Drawing for the job (mm, zero at the part's lowest x, y, z). A direction names the side the tool comes from. Give positions to 0.01 mm unless a question says otherwise; leave off trailing zeros. Order: outer loops, then holes, each group sorted by start corner. A loop starts at its lowest first (then second) coordinate and runs counter-clockwise, first axis right, second up. Notation, with made-up numbers: (25.5, 51) -> (48.5, 51) arc R9 cw to (48.5, 58) -> close; hole circle Ø7 at (7, 71.5). An arc over 180 degrees is marked (long way). Use a Markdown table: item, result. Add a question column.
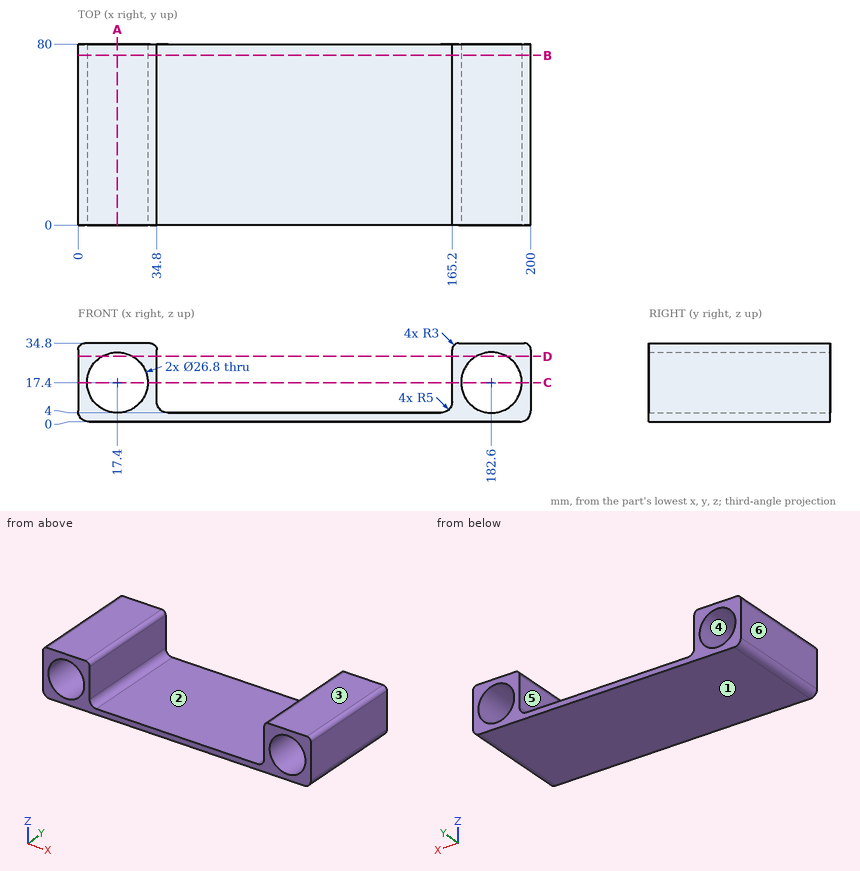
(1) Mould opens along X. For the marked faces 3, 4, 5 and 6 say: released by +X, released by -X, zero draft, split by the parting line, or undercut.
(2) Tool access for the marked faces 1 and 2: list every direction of +Z, -Z, +X, -X, +Y, -Y with a clear straight run to the whole face (end or side of a thin tool).
(3) Band-saw the part on B-B on y = 75. Give the cut face in (x, z).
(4) Band-saw the part on D-D on z = 29. Give the cut face in (x, y).
(5) Band-saw the part on C-C on z = 17.4. Give the cut face in (x, y).
(6) Band-saw the part on A-A on x = 17.4. Give the cut face in (y, z).
(7) Pin check, flat tip, straight feed: pin 1 Ø3 at (x, y) = (44, 20) entering from +Z. Stop position of the tip, or through.
(8) Wall check: probe 1 along X at (y, z) = (4, 17.5); probe 2 along Z at (x, y) = (17, 54); probe 3 along X at (y, z) = (37, 27.5). Give the ranges that are in metal, low to high.
Response:
| question | item | result |
|---|---|---|
| 1 | face 3 | zero draft |
| 1 | face 4 | undercut |
| 1 | face 5 | undercut |
| 1 | face 6 | released by -X |
| 2 | face 1 | -Z, +X, -X, +Y, -Y |
| 2 | face 2 | +Z, +Y, -Y |
| 3 | outline | (0, 5) arc R5 ccw to (5, 0) -> (195, 0) arc R5 ccw to (200, 5) -> (200, 31.8) arc R3 ccw to (197, 34.8) -> (168.2, 34.8) arc R3 ccw to (165.2, 31.8) -> (165.2, 9) arc R5 cw to (160.2, 4) -> (39.8, 4) arc R5 cw to (34.8, 9) -> (34.8, 31.8) arc R3 ccw to (31.8, 34.8) -> (3, 34.8) arc R3 ccw to (0, 31.8) -> close; hole circle Ø26.8 at (17.4, 17.4); hole circle Ø26.8 at (182.6, 17.4) |
| 4 | outline | (0, 0) -> (10.69, 0) -> (10.69, 80) -> (0, 80) -> close; (24.11, 0) -> (34.8, 0) -> (34.8, 80) -> (24.11, 80) -> close; (165.2, 0) -> (175.89, 0) -> (175.89, 80) -> (165.2, 80) -> close; (189.31, 0) -> (200, 0) -> (200, 80) -> (189.31, 80) -> close |
| 5 | outline | (0, 0) -> (4, 0) -> (4, 80) -> (0, 80) -> close; (30.8, 0) -> (34.8, 0) -> (34.8, 80) -> (30.8, 80) -> close; (165.2, 0) -> (169.2, 0) -> (169.2, 80) -> (165.2, 80) -> close; (196, 0) -> (200, 0) -> (200, 80) -> (196, 80) -> close |
| 6 | outline | (0, 0) -> (80, 0) -> (80, 4) -> (0, 4) -> close; (0, 30.8) -> (80, 30.8) -> (80, 34.8) -> (0, 34.8) -> close |
| 7 | pin 1 | stops at z = 4 |
| 8 | probe 1 | x = 0 to 4, 30.8 to 34.8, 165.2 to 169.2, 196 to 200 |
| 8 | probe 2 | z = 0 to 4.01, 30.79 to 34.8 |
| 8 | probe 3 | x = 0 to 8.59, 26.21 to 34.8, 165.2 to 173.79, 191.41 to 200 |
